Read the model definition and answer for the solid it produces. Units are mm, in the model's axes. A direction names the side the tool comes from. Coordinates: 2 decimals unless noted, no trailing zeros. Write each loop counter-clockwise with the first axis right and the second up, starting at its lowest first coordinate (ties: lowest second). Pieces come first, ordered by that corner, then holes. Notation, with made-up numbers: (28.5, 11.25) - (83.5, 11.25) arc R27 ccw to (83.5, 29.25) - close; hole circle Ø8 at (67.5, -39.5). An arc over 180 degrees is marked (long way). Use a Markdown table: item, result.
from build123d import *

# Parameters (mm, degrees)
SKETCH1_R                                           = 30
BOSS_EXTRUDE1_DEPTH                                 = 10
CBORE_FOR_M6_HEX_SOCKET_HEAD_CAP_SCREW1_D           = 6.6
CBORE_FOR_M6_HEX_SOCKET_HEAD_CAP_SCREW1_CBORE_D     = 11
CBORE_FOR_M6_HEX_SOCKET_HEAD_CAP_SCREW1_CBORE_DEPTH = 6.4
CUT_EXTRUDE1_START                                  = -7
CUT_EXTRUDE1_DEPTH                                  = 7
CIRPATTERN1_COUNT                                   = 4
FILLET1_R                                           = 3


with BuildPart() as part:
    # Sketch1 → Boss-Extrude1 (new body)
    with BuildSketch(Plane(origin=(0, 0, 0), x_dir=(1, 0, 0), z_dir=(0, 1, 0))):
        with Locations(Location((0, 0, 0), (0, 0, 270))):
            Circle(SKETCH1_R)
    extrude(amount=BOSS_EXTRUDE1_DEPTH)

    # CBORE for M6 Hex Socket Head Cap Screw1 (through all)
    with Locations(Plane(origin=(0, 10, 0), x_dir=(1, 0, 0), z_dir=(0, 1, 0))):
        with Locations((14.142135624, -14.142135624), (14.142135624, 14.142135624), (-14.142135624, 14.142135624), (-14.142135624, -14.142135624)):
            CounterBoreHole(CBORE_FOR_M6_HEX_SOCKET_HEAD_CAP_SCREW1_D / 2, CBORE_FOR_M6_HEX_SOCKET_HEAD_CAP_SCREW1_CBORE_D / 2, CBORE_FOR_M6_HEX_SOCKET_HEAD_CAP_SCREW1_CBORE_DEPTH)

    # Sketch4 → Cut-Extrude1 (cut)
    with BuildSketch(Plane(origin=(0, 10, 0), x_dir=(1, 0, 0), z_dir=(0, 1, 0)).offset(CUT_EXTRUDE1_START)):
        with BuildLine():
            ThreePointArc((4.592201188, -11.08655439), (0, -12), (-4.592201188, -11.08655439))
            Line((-4.592201188, -11.08655439), (-11.480502971, -27.716385975))
            ThreePointArc((-11.480502971, -27.716385975), (0, -30), (11.480502971, -27.716385975))
            Line((11.480502971, -27.716385975), (4.592201188, -11.08655439))
        make_face()
    cut_extrude1 = extrude(amount=CUT_EXTRUDE1_DEPTH, mode=Mode.SUBTRACT)

    # Sketch6 → M3 Tapped Hole1 (revolve, cut)
    with BuildSketch(Plane(origin=(0, 7, 12), x_dir=(0, -1, 0), z_dir=(1, 0, 0))):
        Polygon((0, 0), (0, 12.751075774), (1.25, 12), (1.25, 0), align=None)
    m3_tapped_hole1 = revolve(axis=Axis((0, 7, 18.35), (0, 0, -1)), mode=Mode.SUBTRACT)

    # CirPattern1: Cut-Extrude1, M3 Tapped Hole1 ×4 about axis
    cirpattern1_axis = Axis((0, 10, 0), (0, 1, 0))
    add([cut_extrude1.rotate(cirpattern1_axis, i * 360 / CIRPATTERN1_COUNT) for i in range(1, CIRPATTERN1_COUNT)], mode=Mode.SUBTRACT)
    add([m3_tapped_hole1.rotate(cirpattern1_axis, i * 360 / CIRPATTERN1_COUNT) for i in range(1, CIRPATTERN1_COUNT)], mode=Mode.SUBTRACT)

    # Fillet1
    fillet1_edges = [part.edges().sort_by_distance(p)[0] for p in [
        (-4.592201188, 6.5, 11.08655439),
        (4.592201188, 6.5, 11.08655439),
        (4.592201188, 6.5, -11.08655439),
        (-4.592201188, 6.5, -11.08655439),
        (-11.08655439, 6.5, -4.592201188),
        (-11.08655439, 6.5, 4.592201188),
        (11.08655439, 6.5, 4.592201188),
        (11.08655439, 6.5, -4.592201188),
    ]]
    fillet(fillet1_edges, radius=FILLET1_R)


solid = part.part
(1) The mould has two halves that part along Z. Classify faces 1 (the flat face through (-20.55, 6.45, -8.51)), 2 (the cylindrical face through (0.38, 5.81, -6.08)), 3 (the cylindrical face through (-26.615, 3.819, 13.843)): pulls with the +Z half, pulls with the -Z half, needs draft (parallel to the pull), parting line crosses it, or undercut.
Report:
| item | result |
|---|---|
| face 1 | undercut |
| face 2 | needs draft |
| face 3 | parting line crosses it |
(2) Straight lines are drawn through the part: L1, parallel to Z at x = -15, y = 9.25; L2, parallel to Y at x = 0, z = -5; L3, parallel to Z at x = 13, y = 3.75. For each, find the intervals that lie inside material, in ascending order.
Report:
| item | result |
|---|---|
| L1 | z = -25.98 to -19.57, -8.71 to -6.21, 6.21 to 8.71, 19.57 to 25.98 |
| L2 | y = 0 to 5.75, 8.25 to 10 |
| L3 | z = -27.04 to -19.52, -8.76 to -5.31, 5.31 to 8.76, 19.52 to 27.04 |
(3) Each of these flat-tipped pins is pushed along its axis until it touches: P1, Ø5.5, axis at x = -12, z = 15, coming from the +Y side; P2, Ø5, axis at x = -4, y = 2, coming from the +Z side; P3, Ø2, axis at y = 5, z = 3.5, coming from the +X side; P4, Ø4, axis at x = -14.14, z = 14.14, coming from the -Y side. Where does it stop, or does it pass through?
Report:
| item | result |
|---|---|
| P1 | stops at y = 3.6 |
| P2 | stops at z = 29.96 |
| P3 | stops at x = 12.22 |
| P4 | passes through |
(4) A cutting plane is placed at B-B, the plane z = 16.5. Write down the section's boundary in (x, y).
Report:
| item | result |
|---|---|
| outline | (-25.05, 0) - (-16.45, 0) - (-16.45, 3.6) - (-19.11, 3.6) - (-19.11, 10) - (-25.05, 10) - close; (-11.83, 0) - (11.83, 0) - (11.83, 3.6) - (9.17, 3.6) - (9.17, 10) - (6.83, 10) - (6.83, 3) - (-6.83, 3) - (-6.83, 10) - (-9.17, 10) - (-9.17, 3.6) - (-11.83, 3.6) - close; (16.45, 0) - (25.05, 0) - (25.05, 10) - (19.11, 10) - (19.11, 3.6) - (16.45, 3.6) - close |
(5) For faces 4 (the cylindrical face through (-11.99, 5.67, -0.48)), 5 (the flat face through (17, 3.6, -12)), 6 (the cylindrical face through (0.542, 5.673, 11.988)), determine the directions among +Z, -Z, +X, -X, +Y, -Y from which every point of the face is accessible in a straight line to the end or side of a thin tool.
Report:
| item | result |
|---|---|
| face 4 | -X, +Y |
| face 5 | +Y |
| face 6 | +Z, +Y |
(6) A cutting plane is placed at D-D, the plane x = 22. Write down the section's boundary in (y, z).
Report:
| item | result |
|---|---|
| outline | (0, -20.4) - (10, -20.4) - (10, -9.11) - (3, -9.11) - (3, 9.11) - (10, 9.11) - (10, 20.4) - (0, 20.4) - close |
(7) A cutting plane is placed at C-C, the plane y = 4.5. Write down the section's boundary in (x, z), and give its area (3 significant figures).
Report:
| item | result |
|---|---|
| outline | (-27.72, -11.48) arc R30 ccw to (-11.48, -27.72) - (-5.62, -13.58) arc R3 cw to (-2.28, -11.78) arc R12 ccw to (2.28, -11.78) arc R3 cw to (5.62, -13.58) - (11.48, -27.72) arc R30 ccw to (27.72, -11.48) - (13.58, -5.62) arc R3 cw to (11.78, -2.28) arc R12 ccw to (11.78, 2.28) arc R3 cw to (13.58, 5.62) - (27.72, 11.48) arc R30 ccw to (11.48, 27.72) - (5.62, 13.58) arc R3 cw to (2.28, 11.78) arc R12 ccw to (-2.28, 11.78) arc R3 cw to (-5.62, 13.58) - (-11.48, 27.72) arc R30 ccw to (-27.72, 11.48) - (-13.58, 5.62) arc R3 cw to (-11.78, 2.28) arc R12 ccw to (-11.78, -2.28) arc R3 cw to (-13.58, -5.62) - close; hole circle Ø11 at (-14.14, -14.14); hole circle Ø11 at (-14.14, 14.14); hole circle Ø11 at (14.14, -14.14); hole circle Ø11 at (14.14, 14.14) |
| area | 1,270 mm² |
(8) A cutting plane is placed at A-A, the plane x = -3.5. Write down the section's boundary in (y, z), and give its area (3 significant figures).
Report:
| item | result |
|---|---|
| outline | (0, -29.8) - (3, -29.8) - (3, -11.8) - (10, -11.8) - (10, 11.8) - (3, 11.8) - (3, 29.8) - (0, 29.8) - close; hole circle Ø2.5 at (7, 0) |
| area | 339 mm² |
